Answer from the drawing. Dimensions are ordinates in mm from the lowest x, y and z of the part. A direction names the side the tool comes from. Coordinates: 2 decimals unless noted, no trailing zeros. Order: outer loops, then holes, each group sorted by start corner. A loop starts at its lowest first (then second) coordinate and runs counter-clockwise, first axis right, second up. Notation, with made-up numbers: M -36,14 L -15,14 A30 cw -15,42 Z; hole C -1.75,-14.75 d7. An arc over 180 degrees is marked long. Use a Markdown table: item, result.
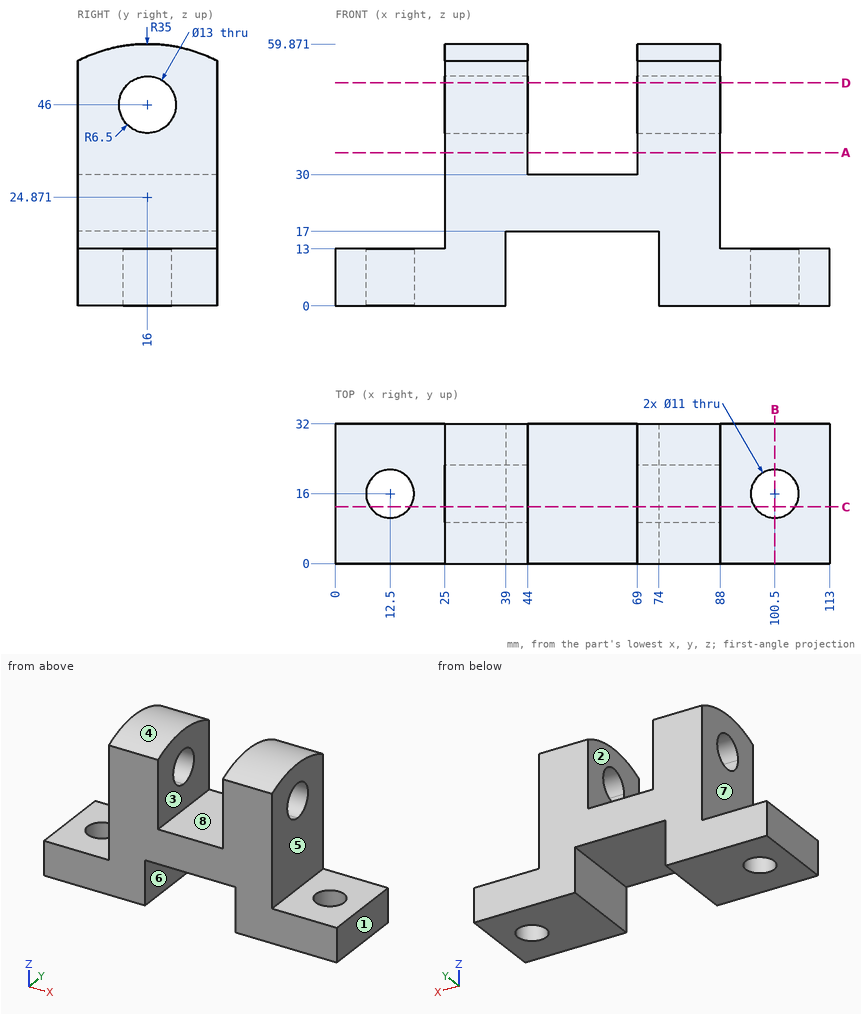
(1) Determine the mould class of the marked faces 1, 2, 3 and 4 for opening direction X: pulls with the +X half, pulls with the -X half, needs draft (parallel to the pull), parting line crosses it, or undercut.
Conclusion:
| item | result |
|---|---|
| face 1 | pulls with the +X half |
| face 2 | undercut |
| face 3 | undercut |
| face 4 | needs draft |
(2) A cutting plane is placed at D-D (z = 51). Determine the outline of the cut face in (x, y).
Conclusion:
| item | result |
|---|---|
| outline | M 25,0 L 44,0 L 44,11.85 L 25,11.85 Z; M 25,20.15 L 44,20.15 L 44,32 L 25,32 Z; M 69,0 L 88,0 L 88,11.85 L 69,11.85 Z; M 69,20.15 L 88,20.15 L 88,32 L 69,32 Z |
(3) A cutting plane is placed at C-C (y = 13). Give the number of separate pieces and of enclosed holes in the cut face, then the cut area to 3 significant figures.
Conclusion:
| item | result |
|---|---|
| separate pieces | 5 |
| enclosed holes | 0 |
| area | 2,400 mm2 |
(4) Straight lines are drawn through the part: L1, parallel to X at y = 15.5, z = 4.5; L2, parallel to Y at x = 100, z = 9; L3, parallel to X at y = 26.5, z = 35.5. For each, find the intervals that lie inside material, in ascending order.
Conclusion:
| item | result |
|---|---|
| L1 | 0 to 7.02, 17.98 to 39, 74 to 95.02, 105.98 to 113 |
| L2 | 0 to 10.52, 21.48 to 32 |
| L3 | 25 to 44, 69 to 88 |
(5) A cutting plane is placed at B-B (x = 100.5). Determine the outline of the cut face in (y, z).
Conclusion:
| item | result |
|---|---|
| outline | M 0,0 L 10.5,0 L 10.5,13 L 0,13 Z; M 21.5,0 L 32,0 L 32,13 L 21.5,13 Z |
(6) Which of the six approach directions +Z, -Z, +X, -X, +Y, -Y give full straight-line access (tool end or side, diameter ignored) to the marked faces 5, 6, 7 and 8?
Conclusion:
| item | result |
|---|---|
| face 5 | +Z, +X, +Y, -Y |
| face 6 | -Z, +Y, -Y |
| face 7 | +Z, -X, +Y, -Y |
| face 8 | +Z, +Y, -Y |
(7) A cutting plane is placed at A-A (z = 35). Determine the outline of the cut face in (x, y), then the cut area to 3 significant figures.
Conclusion:
| item | result |
|---|---|
| outline | M 25,0 L 44,0 L 44,32 L 25,32 Z; M 69,0 L 88,0 L 88,32 L 69,32 Z |
| area | 1,220 mm2 |
(8) Given P1, Ø9, axis at y = 15.5, z = 52, coming from the +X side; P2, Ø12.5, axis at x = 58, y = 13, coming from the +Z side; P3, Ø9.5, axis at y = 13.5, z = 45, coming from the -X side, each flat-ended and moving along its own axis, determine where each tip first touches the part or whether it passes through.
Conclusion:
| item | result |
|---|---|
| P1 | x = 88 |
| P2 | z = 30 |
| P3 | x = 25 |
